Autodesk Fusion 360 part; units mm, degrees
sketch "CF63 Profile" plane through (0, 0, 0) normal (1, 0, 0) x (0, 0, -1)
  line L0 (-38.3816, -1.2) -> (-38.6, -0.6)
  line L1 (-50.25, -30) -> (-50.25, 0)
  line L2 (-38.3816, -1.2) -> (0, -1.2)
  line L3 (-41.85, 0) -> (-41.85, -30)
  line L4 (-41.275, -1.5736) -> (-38.6, -0.6)
  line L5 (-50.25, 0) -> (-41.275, 0)
  line L6 (-41.275, -1.5736) -> (-41.275, 0)
  line L7 (-46.05, 0) -> (-46.05, -30)
  line L8 (0, 0) -> (0, -30)
  line L9 (0, -30) -> (-53, -30)
  line L10 (-53, -30) -> (-53, 0)
  line L11 (-53, 0) -> (-50.25, 0)
  line L12 (-35, -1.2) -> (-35, -30)
  dimension "d1" = 30
  dimension "d2" = 53
  dimension "d3" = 35
revolve "Revolve1" add sketch "CF63 Profile" angle 360 about axis through (0, 0, 0) along (0, -1, 0) contours L0 L2 L3 L4 L5 L6 L9 L12 | L3 L5 L7 L9 | L1 L5 L7 L9 | L1 L9 L10 L11
chamfer "Chamfer1" distance 0.5 angle 45 4 edges at (-32.6315, -1.2, 12.6565) (-32.6315, -30, 12.6565) (-49.4133, 0, 19.1656) (-49.4133, -30, 19.1656)
sketch "Sketch2" plane through (0, 0, 0) normal (0, 1, 0) x (-1, 0, 0)
  circle A0 centre (0, 0) radius 41.275
  circle A1 centre (0, 0) radius 52.5
  point P0 (0, 46.05)
hole "Hole1" at (0, 0, 46.05) direction (0, -1, 0) diameter 6.78 depth 15 tip angle 118
pattern_circular "C-Pattern2" count 8 over 360 about axis through (0, 1.75, 0) along (0, 1, 0) of "Hole1"
Can you work these out from the model? Positions are in its coordinate system, mm. A direction names the side the tool comes from. Round coordinates to 2 decimals unless told otherwise and drop trailing zeros. Order: outer loops, then holes, each group sorted by start corner. A loop starts at its lowest first (then second) coordinate and runs counter-clockwise, first axis right, second up.
(1) If we section it at A-A (y = -9): Count the separate pieces of the cut face and the enclosed holes in it, plus the area to 3 significant figures.
Results are:
separate pieces: 1
enclosed holes: 9
area: 4,690 mm2
(2) On a 3-axis mill with a long thin cutter (end or side, diameter ignored), from which of +Z, -Z, +X, -X, +Y, -Y can I reach the whole of each face in a straight line? I mean faces 1 (the face through (11, -30, 34)), 2 (the face through (-32.12, -7.6, -29.2)). Say none if no direction works.
Results are:
face 1: +Z, -Z, +X, -X, -Y
face 2: +Y
(3) If we section it at B-B (y = -19): Please give me the cut outline in (x, z), plus the area to 3 significant figures.
Results are:
outline: circle Ø106 at (0, 0); hole circle Ø70 at (0, 0)
area: 4,980 mm2
(4) If I drill on L1, parallel to Z at x = 0, y = -18.5; L2, parallel to Z at x = -1, y = -12; L3, parallel to X at y = -18, z = -13, over which ranges is the centre line in solid material (lowest first)?
Results are:
L1: z = -53 to -35, 35 to 53
L2: z = -52.99 to -49.29, -42.81 to -34.99, 34.99 to 42.81, 49.29 to 52.99
L3: x = -51.38 to -32.5, 32.5 to 51.38
(5) We'd pull the mould along X, two halves only. Please class faces 3 (the face through (21, -16, -28)), 4 (the face through (39, 0, 15)): +X half, -X half, draft (parallel to the pull), parting line (faces both ways), or undercut.
Results are:
face 3: undercut
face 4: draft
(6) I'm going to push flat-ended pins straight in: pin 1 (1 mm diameter, centred on x = 21.5, y = -20, fed in from +Z); pin 2 (8 mm diameter, centred on y = -14.5, z = -17, fed in from -X); pin 3 (2 mm diameter, centred on y = -17.5, z = -34.5, fed in from -X). Where does each tip first touch, or does it pass through?
Results are:
pin 1: stops at z = 48.66
pin 2: stops at x = -51.38
pin 3: stops at x = -41.07
